Model file for the job. Use its own axes, mm. Face numbers are marked on the shaded views. A direction names the side the tool comes from. Give positions to 0.01 mm unless a question says otherwise; leave off trailing zeros. Order: outer loops, then holes, each group sorted by start corner. A loop starts at its lowest first (then second) coordinate and runs counter-clockwise, first axis right, second up. Notation, with made-up numbers: M 27,83.5 L 40,83.5 A32 ccw 40,114.5 Z; hole C 51,43.25 d9. An arc over 180 degrees is marked long. Return JSON: item names as keys, results as strings. Group by question number.
1. Slice it at D-D on y = 53.5. List the corners of the cut face in (x, z).
2. 3-axis set-ups, long thin cutter, end or side, ignore diameter. For the marked faces 4, 5 and 6: which of +Z, -Z, +X, -X, +Y, -Y reach the whole face in a straight line?
3. Two-plate mould, pull along X, no slides. Class the marked faces 1, 2 and 3: released by +X, released by -X, zero draft, split by the parting line, or undercut.
4. Slice it at C-C on x = 2. List the corners of the cut face in (y, z), then the cut area to 3 significant figures.
5. Slice it at B-B on y = 68. List the corners of the cut face in (x, z).
6. Wall check: probe 1 along X at (y, z) = (68, 0.8); probe 2 along Y at (x, z) = (48, 0.95); probe 3 along X at (y, z) = (24.5, 2.25). Give the ranges that are in metal, low to high. Write a range as [from, to].
7. Pin check, flat tips, straight feed: pin 1 (4.5 mm diameter, centred on x = 2, y = 2, fed in from -Z); pin 2 (1 mm diameter, centred on y = 61, z = 1, fed in from -X); pin 3 (5.5 mm diameter, centred on x = 48, y = 68, fed in from +Z). Stop position of each tip, or through.
8. Slice it at A-A on x = 48. List the corners of the cut face in (y, z), then the cut area to 3 significant figures.
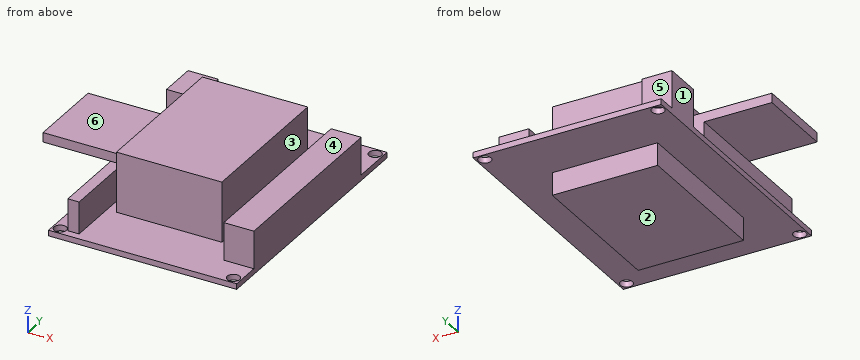
from build123d import *

# Parameters (mm, degrees)
SKETCH1_W               = 50
SKETCH1_H               = 70
SKETCH1_R               = 1.65
MAIN_PROTOBOARD_DEPTH   = 1.5
SCREW_TERMINALS_START   = 1.5
SKETCH1_3_W             = 8
SKETCH1_3_H             = 50
SKETCH1_3_H_2           = 10
SCREW_TERMINALS_DEPTH   = 10
MCU_START               = 1.5
SKETCH1_5_W             = 28
SKETCH1_5_H             = 40
MCU_DEPTH               = 16
SKETCH1_6_W             = 3
SKETCH1_6_H             = 41
DUPONT_CONNECTORS_DEPTH = 10
CAN_TRANSCEIVER_START   = 10
SKETCH1_7_W             = 14
SKETCH1_7_H             = 21
SKETCH1_7_W_2           = 4
SKETCH1_7_W_3           = 3
CAN_TRANSCEIVER_DEPTH   = 2.5
SKETCH1_8_W             = 28
SKETCH1_8_H             = 40
WIRE_CLEARANCE_DEPTH    = 6


with BuildPart() as part:
    # Sketch1 → Main-Protoboard (new body)
    with BuildSketch(Plane.XY):
        with Locations((25, 35)):
            Rectangle(SKETCH1_W, SKETCH1_H)
        with Locations((2, 2)):
            Circle(SKETCH1_R, mode=Mode.SUBTRACT)
        with Locations((48, 2)):
            Circle(SKETCH1_R, mode=Mode.SUBTRACT)
        with Locations((2, 68)):
            Circle(SKETCH1_R, mode=Mode.SUBTRACT)
        with Locations((48, 68)):
            Circle(SKETCH1_R, mode=Mode.SUBTRACT)
    extrude(amount=MAIN_PROTOBOARD_DEPTH)

    # Sketch1<3> → Screw-Terminals (add)
    with BuildSketch(Plane.XY.offset(SCREW_TERMINALS_START)):
        with Locations((46, 33)):
            Rectangle(SKETCH1_3_W, SKETCH1_3_H)
        with Locations((4, 60)):
            Rectangle(SKETCH1_3_W, SKETCH1_3_H_2)
    extrude(amount=SCREW_TERMINALS_DEPTH)

    # Sketch1<5> → MCU (add)
    with BuildSketch(Plane.XY.offset(MCU_START)):
        with Locations((23.5, 35)):
            Rectangle(SKETCH1_5_W, SKETCH1_5_H)
    extrude(amount=MCU_DEPTH)

    # Sketch1<6> → Dupont-Connectors (add)
    with BuildSketch(Plane.XY):
        with Locations((5.5, 22.5)):
            Rectangle(SKETCH1_6_W, SKETCH1_6_H)
    extrude(amount=DUPONT_CONNECTORS_DEPTH)

    # Sketch1<7> → Can-Transceiver (add)
    with BuildSketch(Plane.XY.offset(CAN_TRANSCEIVER_START)):
        with Locations((-7, 32.5)):
            Rectangle(SKETCH1_7_W, SKETCH1_7_H)
        with Locations((2, 32.5)):
            Rectangle(SKETCH1_7_W_2, SKETCH1_7_H)
        with Locations((5.5, 32.5)):
            Rectangle(SKETCH1_7_W_3, SKETCH1_7_H)
    extrude(amount=CAN_TRANSCEIVER_DEPTH)

    # Sketch1<8> → Wire-Clearance (add)
    with BuildSketch(Plane.XY):
        with Locations((23.5, 35)):
            Rectangle(SKETCH1_8_W, SKETCH1_8_H)
    extrude(amount=-WIRE_CLEARANCE_DEPTH)


solid = part.part
Result:
{
 "1": {"outline": "M 0,0 L 9.5,0 L 9.5,-6 L 37.5,-6 L 37.5,0 L 50,0 L 50,11.5 L 42,11.5 L 42,1.5 L 37.5,1.5 L 37.5,17.5 L 9.5,17.5 L 9.5,1.5 L 0,1.5 Z"},
 "2": {"face 4": "+Z, +X, +Y, -Y", "face 5": "+Z, +X, -X, +Y", "face 6": "+Z, -X, +Y, -Y"},
 "3": {"face 1": "released by -X", "face 2": "zero draft", "face 3": "undercut"},
 "4": {"outline": "M 0,0 L 0.35,0 L 0.35,1.5 L 0,1.5 Z; M 3.65,0 L 66.35,0 L 66.35,1.5 L 65,1.5 L 65,11.5 L 55,11.5 L 55,1.5 L 3.65,1.5 Z; M 22,10 L 43,10 L 43,12.5 L 22,12.5 Z; M 69.65,0 L 70,0 L 70,1.5 L 69.65,1.5 Z", "area": "248 mm2"},
 "5": {"outline": "M 0,0 L 0.35,0 L 0.35,1.5 L 0,1.5 Z; M 3.65,0 L 46.35,0 L 46.35,1.5 L 3.65,1.5 Z; M 49.65,0 L 50,0 L 50,1.5 L 49.65,1.5 Z"},
 "6": {"probe 1": "x = [0, 0.35], [3.65, 46.35], [49.65, 50]", "probe 2": "y = [0, 0.35], [3.65, 66.35], [69.65, 70]", "probe 3": "x = [4, 7], [9.5, 37.5], [42, 50]"},
 "7": {"pin 1": "stops at z = 0", "pin 2": "stops at x = 0", "pin 3": "stops at z = 1.5"},
 "8": {"outline": "M 0,0 L 0.35,0 L 0.35,1.5 L 0,1.5 Z; M 3.65,0 L 66.35,0 L 66.35,1.5 L 58,1.5 L 58,11.5 L 8,11.5 L 8,1.5 L 3.65,1.5 Z; M 69.65,0 L 70,0 L 70,1.5 L 69.65,1.5 Z", "area": "595 mm2"}
}
